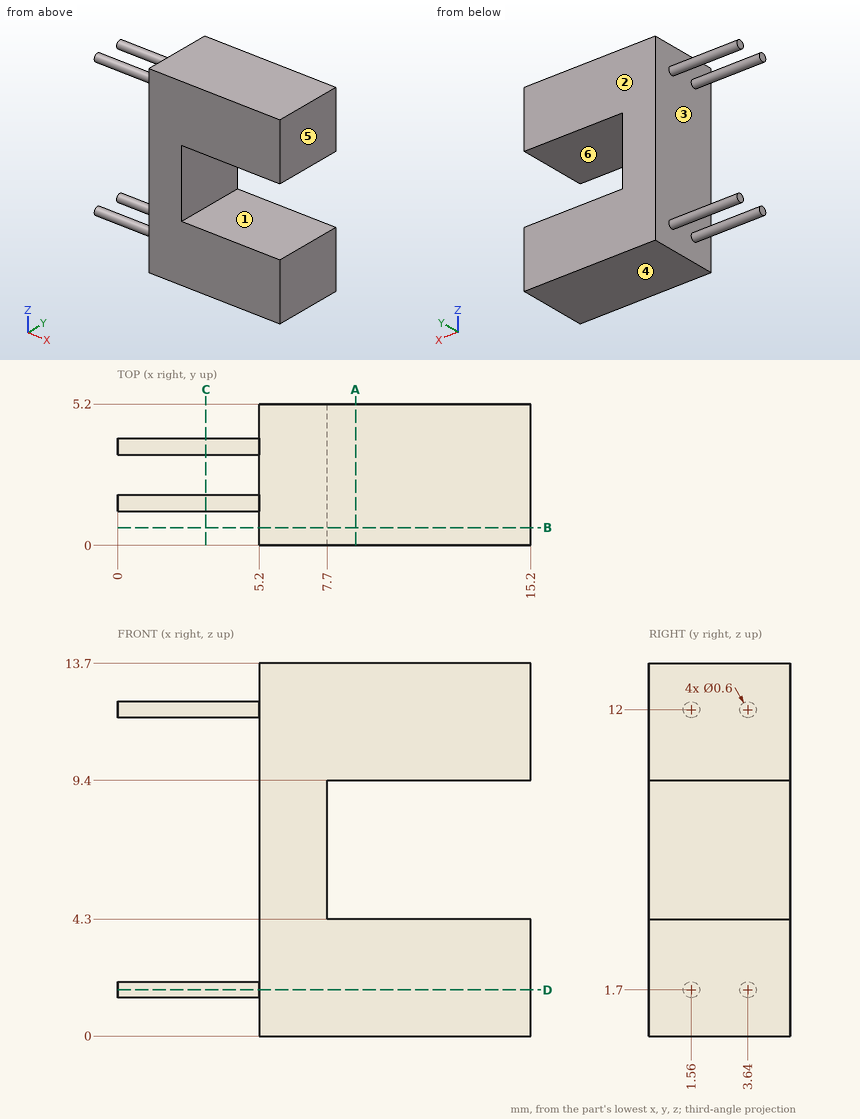
Geometry check sheet. Reference: drawing and pictorial views, mm from the part's lowest x, y, z. A direction names the side the tool comes from. Coordinates: 2 decimals unless noted, no trailing zeros. Order: outer loops, then holes, each group sorted by start corner. A loop starts at its lowest first (then second) coordinate and runs counter-clockwise, first axis right, second up.
1. Scan lines: line 1 (Z direction, x = 12.5, y = 4.5); line 2 (X direction, y = 1.35, z = 7.5); line 3 (X direction, y = 4.8, z = 12.75). Record each from-to range of solid material in increasing order.
Results found:
line 1: z = 0 to 4.3, 9.4 to 13.7
line 2: x = 5.2 to 7.7
line 3: x = 5.2 to 15.2
2. Sectioned sample at A-A, the plane x = 8.75. Record the cut outline in (y, z).
Results found:
outline: (0, 0) - (5.2, 0) - (5.2, 4.3) - (0, 4.3) - close; (0, 9.4) - (5.2, 9.4) - (5.2, 13.7) - (0, 13.7) - close
3. Sectioned sample at C-C, the plane x = 3.25. Record the cut outline in (y, z).
Results found:
outline: circle Ø0.6 at (1.56, 1.7); circle Ø0.6 at (1.56, 12); circle Ø0.6 at (3.64, 1.7); circle Ø0.6 at (3.64, 12)
4. Release check for a two-part mould opening along Z. For the marked faces 3, 4, 5 and 6 record: +Z half, -Z half, draft (parallel to the pull), parting line (faces both ways), or undercut.
Results found:
face 3: undercut
face 4: -Z half
face 5: draft
face 6: undercut
5. Set-up check for the marked faces 1 and 2: record each of +Z, -Z, +X, -X, +Y, -Y from which the full face is reachable in a straight line by a thin tool's end or side.
Results found:
face 1: +X, +Y, -Y
face 2: +Z, -Z, +X, -X, +Y
6. Sectioned sample at B-B, the plane y = 0.65. Record the cut outline in (x, z), and give its area (4 significant figures).
Results found:
outline: (5.2, 0) - (15.2, 0) - (15.2, 4.3) - (7.7, 4.3) - (7.7, 9.4) - (15.2, 9.4) - (15.2, 13.7) - (5.2, 13.7) - close
area: 98.75 mm2
7. Sectioned sample at D-D, the plane z = 1.7. Record the cut outline in (x, y), and give its area (3 significant figures).
Results found:
outline: (0, 1.26) - (5.2, 1.26) - (5.2, 0) - (15.2, 0) - (15.2, 5.2) - (5.2, 5.2) - (5.2, 3.94) - (0, 3.94) - (0, 3.34) - (5.2, 3.34) - (5.2, 1.86) - (0, 1.86) - close
area: 58.2 mm2
